from build123d import *

# Parameters (mm, degrees)
BOSS_EXTRUDE1_DEPTH = 50
SKETCH3_R           = 3
CUT_EXTRUDE1_DEPTH  = 54.909646632


with BuildPart() as part:
    # Sketch2 → Boss-Extrude1 (new body)
    with BuildSketch(Plane.XY):
        with BuildLine():
            Line((-17.5, -11.928580859), (-7.937253933, -11.928580859))
            ThreePointArc((-7.937253933, -11.928580859), (0, -18.928580859), (7.937253933, -11.928580859))
            Line((7.937253933, -11.928580859), (17.5, -11.928580859))
            Line((17.5, -11.928580859), (17.5, -21.928580859))
            Line((17.5, -21.928580859), (-17.5, -21.928580859))
            Line((-17.5, -21.928580859), (-17.5, -11.928580859))
        make_face()
    extrude(amount=-BOSS_EXTRUDE1_DEPTH)

    # Sketch3 → Cut-Extrude1 (cut, through all)
    with BuildSketch(Plane.XZ.offset(21.928580859)):
        with Locations(Location((12.5, -6, 0), (0, 0, 270))):
            Circle(SKETCH3_R)
        with Locations(Location((-12.5, -6, 0), (0, 0, 90))):
            Circle(SKETCH3_R)
        with Locations(Location((-12.5, -44, 0), (0, 0, 270))):
            Circle(SKETCH3_R)
        with Locations(Location((12.5, -44, 0), (0, 0, 90))):
            Circle(SKETCH3_R)
    extrude(amount=-CUT_EXTRUDE1_DEPTH, mode=Mode.SUBTRACT)


solid = part.part
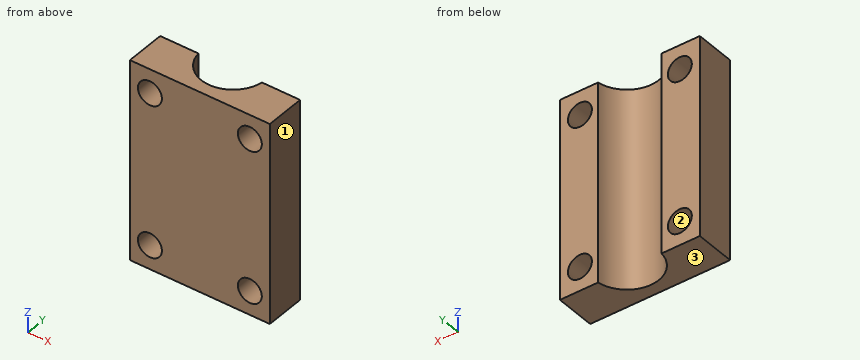
Here's how the part is built. I have some questions about the finished solid (model axes, mm). Face numbers are marked on the shaded views. Coordinates: 2 decimals unless noted, no trailing zeros. Write each loop counter-clockwise with the first axis right and the second up, starting at its lowest first coordinate (ties: lowest second). Pieces come first, ordered by that corner, then holes.
Item 1: I want a section at D-D on y = -17.25. Write out the boundary of the cut face in (x, z).
Item 2: If we mould it in two halves opening along Z, with no side actions, what happens to the marked faces 1, 2 and 3? For each: +Z half, -Z half, draft (parallel to the pull), parting line (faces both ways), or undercut.
Item 3: I want a section at B-B on z = -44. Write out the boundary of the cut face in (x, y).
Item 4: I want a section at A-A on x = 12.5. Write out the boundary of the cut face in (y, z), and give its area (3 significant figures).
Item 5: If I drill on line 1 (X direction, y = -19.5, z = -44); line 2 (Z direction, x = -11.5, y = -21); line 3 (X direction, y = -15, z = -6), over which ranges is the centre line in solid material (lowest first)?
Item 6: I want a section at C-C on y = -20. Write out the boundary of the cut face in (x, z), and give its area (3 significant figures).
Findings below:
1. outline: (-17.5, -50) - (-4.9, -50) - (-4.9, 0) - (-17.5, 0) - close; (4.9, -50) - (17.5, -50) - (17.5, 0) - (4.9, 0) - close; hole circle Ø6 at (-12.5, -44); hole circle Ø6 at (-12.5, -6); hole circle Ø6 at (12.5, -44); hole circle Ø6 at (12.5, -6)
2. face 1: draft
2. face 2: undercut
2. face 3: -Z half
3. outline: (-17.5, -21.93) - (-15.5, -21.93) - (-15.5, -11.93) - (-17.5, -11.93) - close; (-9.5, -21.93) - (9.5, -21.93) - (9.5, -11.93) - (7.94, -11.93) arc R8 cw to (-7.94, -11.93) - (-9.5, -11.93) - close; (15.5, -21.93) - (17.5, -21.93) - (17.5, -11.93) - (15.5, -11.93) - close
4. outline: (-21.93, -50) - (-11.93, -50) - (-11.93, -47) - (-21.93, -47) - close; (-21.93, -41) - (-11.93, -41) - (-11.93, -9) - (-21.93, -9) - close; (-21.93, -3) - (-11.93, -3) - (-11.93, 0) - (-21.93, 0) - close
4. area: 380 mm2
5. line 1: x = -17.5 to -15.5, -9.5 to 9.5, 15.5 to 17.5
5. line 2: z = -50 to -46.83, -41.17 to -8.83, -3.17 to 0
5. line 3: x = -17.5 to -15.5, -9.5 to -6.89, 6.89 to 9.5, 15.5 to 17.5
6. outline: (-17.5, -50) - (17.5, -50) - (17.5, 0) - (-17.5, 0) - close; hole circle Ø6 at (-12.5, -44); hole circle Ø6 at (-12.5, -6); hole circle Ø6 at (12.5, -44); hole circle Ø6 at (12.5, -6)
6. area: 1,640 mm2
